Solid Edge part; units mm, degrees
sketch "Sketch1" plane through (0, 0, 0) normal (0, -1, 0) x (1, 0, 0)
  line L0 (8, 4.6188) -> (0, 9.2376)
  line L1 (0, 9.2376) -> (-8, 4.6188)
  line L2 (-8, 4.6188) -> (-8, -4.6188)
  line L3 (-8, -4.6188) -> (0, -9.2376)
  line L4 (0, -9.2376) -> (8, -4.6188)
  line L5 (8, -4.6188) -> (8, 4.6188)
extrude "Protrusion1" add sketch "Sketch1" along normal mid plane 9.5
sketch "Sketch2" plane through (0, 0, 0) normal (1, 0, 0) x (0, 1, 0)
  line L0 (-4.75, 7.25) -> (-4.2174, 9.2376)
revolve "RevolvedCutout1" cut sketch "Sketch2" angle 360 about axis through (0, 0, 0) along (0, -1, 0) material side at (0, -4.532, 8.2567)
mirror "Mirror1" about plane through (0, 0, 0) normal (0, -1, 0) of "RevolvedCutout1"
hole "孔_7" at (0, -4.75, 0) direction (0, 1, 0) diameter 8.376 end up to next start chamfer 1 start chamfer angle 60 end chamfer 1 end chamfer angle 60
Geometry check sheet. Reference: the model listing, model coordinates, mm. Give positions to 0.01 mm unless a question says otherwise; leave off trailing zeros. Loops run counter-clockwise (first coordinate to the right, second up) from the corner with the lowest first, then second, coordinate; pieces in that order, holes last. Notation, with made-up numbers: M 39.25,70 L 50.25,70 A15 ccw 50.25,77 Z; hole C 55.25,29.5 d4. An arc over 180 degrees is marked long. Write item = value, one per line. Start each with the question number.
1. Section check A-A, the plane z = 0. Enter the section's corners in (x, y), plus the area to 3 significant figures.
2. Draft check along Z on faces 1 (the face through (3.944, 0.064, -6.961)), 2 (the face through (5, -4.75, 2)), 3 (the face through (4.056, 0.064, 6.896)), 4 (the face through (2.83, -0.058, 3.087)). Enter one of: +Z half, -Z half, draft (parallel to the pull), parting line (faces both ways), or undercut.
3. Thickness scan on probe 1 along X at (y, z) = (2, 0); probe 2 along Z at (x, y) = (3, 4.25); probe 3 along X at (y, z) = (-2, -2.25). Record the ranges inside material, lowest first.
4. Section check B-B, the plane y = 2.5. Enter the section's corners in (x, z).
5. Go/stop test with a flat-tipped pin: P1, Ø2, axis at y = 2.5, z = -6.5, coming from the +X side. Record where the tip stops, or that it passes through.
Values follow:
q1.outline = M -8,-4.55 L -7.25,-4.75 L -5.19,-4.75 L -4.19,-4.17 L -4.19,4.17 L -5.19,4.75 L -7.25,4.75 L -8,4.55 Z; M 4.19,-4.17 L 5.19,-4.75 L 7.25,-4.75 L 8,-4.55 L 8,4.55 L 7.25,4.75 L 5.19,4.75 L 4.19,4.17 Z
q1.area = 71.0 mm^2
q2.face_1 = -Z half
q2.face_2 = draft
q2.face_3 = +Z half
q2.face_4 = undercut
q3.probe_1 = -8 to -4.19, 4.19 to 8
q3.probe_2 = -7.51 to -3.11, 3.11 to 7.51
q3.probe_3 = -8 to -3.53, 3.53 to 8
q4.outline = M -8,-4.62 L 0,-9.24 L 8,-4.62 L 8,4.62 L 0,9.24 L -8,4.62 Z; hole C 0,0 d8.38
q5.P1 = 6.47
